Geometry check sheet. Reference: the model listing, model coordinates, mm. Face numbers are marked on the shaded views. A direction names the side the tool comes from. Give positions to 0.01 mm unless a question says otherwise; leave off trailing zeros. Loops run counter-clockwise (first coordinate to the right, second up) from the corner with the lowest first, then second, coordinate; pieces in that order, holes last.
1. Tool access check on the marked faces 1, 2 and 3. Record the directions out of +Z, -Z, +X, -X, +Y, -Y that give a thin tool (end or side, any length) a straight path to the whole face; none if there is none.
2. Go/stop test with flat-tipped pins: pin 1 Ø1 at (x, z) = (-15.5, 32.5) entering from +Y; pin 2 Ø3 at (y, z) = (6.5, 7) entering from +X; pin 3 Ø11 at (y, z) = (23, 45) entering from +X. Record where each tip stops, or that it passes through.
3. Cross-section at A-A, the plane z = 56. Record the cut outline in (x, y), plus the area to 3 significant figures.
4. Cross-section at D-D, the plane y = 18.25. Record the cut outline in (x, z), plus the area to 3 significant figures.
5. Cross-section at C-C, the plane z = 6. Record the cut outline in (x, y), plus the area to 3 significant figures.
6. Material ranges on L1, parallel to Y at x = 15, z = 44; L2, parallel to Z at x = 16.5, y = 20.5; L3, parallel to Z at x = 14.5, y = 14.75, recorded low to high.
7. Cross-section at B-B, the plane y = 10.25. Record the cut outline in (x, z).
from build123d import *

# Parameters (mm, degrees)
BOSS_EXTRUDE1_DEPTH = 60
SKETCH3_W           = 15
SKETCH3_H           = 36
BOSS_EXTRUDE2_DEPTH = 10
SKETCH4_W           = 10
SKETCH4_H           = 10
CUT_EXTRUDE2_DEPTH  = 40


with BuildPart() as part:
    # Sketch1 → Boss-Extrude1 (new body)
    with BuildSketch(Plane.XY):
        Polygon((-22.044198895, 13.662983425), (-22.044198895, -4.337016575), (22.955801105, -4.337016575), (22.955801105, 15.662983425), (7.955801105, 15.662983425), (7.955801105, 25.662983425), (-10.044198895, 25.662983425), align=None)
    extrude(amount=BOSS_EXTRUDE1_DEPTH)

    # Sketch3 → Boss-Extrude2 (add)
    with BuildSketch(Plane(origin=(0, 15.662983425, 0), x_dir=(1, 0, 0), z_dir=(0, 1, 0))):
        with Locations((15.455801105, -18)):
            Rectangle(SKETCH3_W, SKETCH3_H)
    extrude(amount=BOSS_EXTRUDE2_DEPTH)

    # Sketch4 → Cut-Extrude2 (cut)
    with BuildSketch(Plane(origin=(0, 25.662983425, 0), x_dir=(1, 0, 0), z_dir=(0, 1, 0))):
        with Locations((17.955801105, -5)):
            Rectangle(SKETCH4_W, SKETCH4_H)
    extrude(amount=-CUT_EXTRUDE2_DEPTH, mode=Mode.SUBTRACT)


solid = part.part
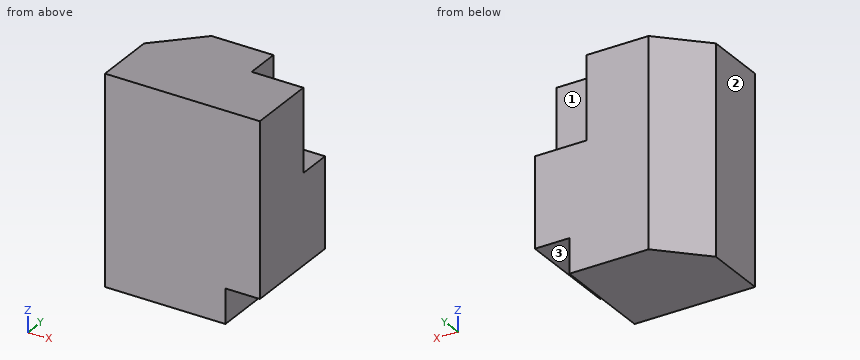
Result:
1. face 1: +Z, +X, +Y
1. face 2: +Z, -Z, -X, +Y, -Y
1. face 3: -Z, +X, +Y, -Y
2. pin 1: stops at y = 20.71
2. pin 2: stops at x = 12.96
2. pin 3: stops at x = 7.96
3. outline: (-22.04, -4.34) - (22.96, -4.34) - (22.96, 15.66) - (7.96, 15.66) - (7.96, 25.66) - (-10.04, 25.66) - (-22.04, 13.66) - close
3. area: 1,130 mm2
4. outline: (-17.46, 0) - (12.96, 0) - (12.96, 10) - (22.96, 10) - (22.96, 36) - (7.96, 36) - (7.96, 60) - (-17.46, 60) - close
4. area: 1,960 mm2
5. outline: (-22.04, -4.34) - (12.96, -4.34) - (12.96, 25.66) - (-10.04, 25.66) - (-22.04, 13.66) - close
5. area: 978 mm2
6. L1: y = -4.34 to 15.66
6. L2: z = 10 to 36
6. L3: z = 10 to 60
7. outline: (-22.04, 0) - (12.96, 0) - (12.96, 10) - (22.96, 10) - (22.96, 60) - (-22.04, 60) - close
